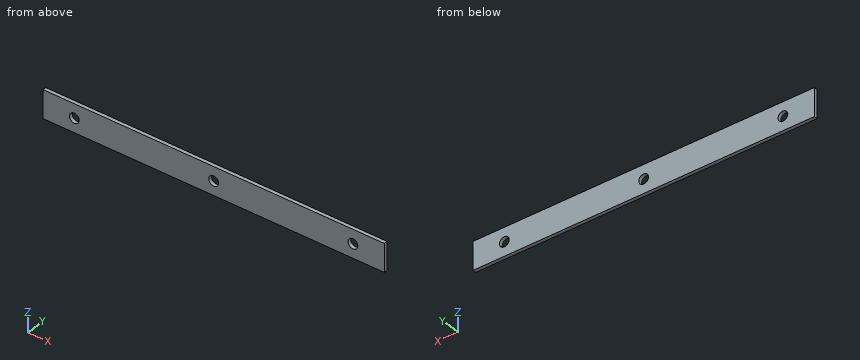
```python
from build123d import *

# Parameters (mm, degrees)
SKETCH1_W            = 245
SKETCH1_H            = 20
BASE_FLANGE1_DEPTH   = 2.5
SKETCH6_R            = 3.5
CUT_EXTRUDE1_DEPTH   = 10
LPATTERN1_COUNT      = 6
LPATTERN1_PITCH      = 146
LPATTERN1_COUNT_DIR2 = 6
LPATTERN1_PITCH_DIR2 = 146
LPATTERN2_COUNT      = 2
LPATTERN2_PITCH      = 100
LPATTERN2_COL_COUNT  = 2
LPATTERN2_COL_PITCH  = 100


# Sheet-metal steps are written as plain solids
with BuildPart() as part:
    # Sketch1 → Base-Flange1 (new body)
    with BuildSketch(Plane(origin=(0, 0, 0), x_dir=(1, 0, 0), z_dir=(0, 1, 0))):
        Rectangle(SKETCH1_W, SKETCH1_H)
    extrude(amount=-BASE_FLANGE1_DEPTH)

    # Sketch6 → Cut-Extrude1 (cut)
    with BuildSketch(Plane(origin=(0, 0, 0), x_dir=(1, 0, 0), z_dir=(0, 1, 0))):
        with Locations(Location((0, 0, 0), (0, 0, 270))):
            Circle(SKETCH6_R)
    cut_extrude1 = extrude(amount=-CUT_EXTRUDE1_DEPTH, mode=Mode.SUBTRACT)

    # LPattern1: Cut-Extrude1 6 × 6
    with Locations(*[Vector(-1, 0, 0) * (i * LPATTERN1_PITCH) + Vector(1, 0, 0) * (j * LPATTERN1_PITCH_DIR2) for i in range(LPATTERN1_COUNT) for j in range(LPATTERN1_COUNT_DIR2) if (i, j) != (0, 0)]):
        add(cut_extrude1, mode=Mode.SUBTRACT)

    # LPattern2: Cut-Extrude1 ×2
    with Locations(*[(-i * LPATTERN2_PITCH, 0, 0) for i in range(1, LPATTERN2_COUNT)]):
        add(cut_extrude1, mode=Mode.SUBTRACT)

    # LPattern2 col: Cut-Extrude1 ×2
    with Locations(*[(i * LPATTERN2_COL_PITCH, 0, 0) for i in range(1, LPATTERN2_COL_COUNT)]):
        add(cut_extrude1, mode=Mode.SUBTRACT)


solid = part.part
```
CAD build for the part. Positions are in the model's coordinates, mm. Coordinates: 2 decimals unless noted, no trailing zeros. Write each loop counter-clockwise with the first axis right and the second up, starting at its lowest first coordinate (ties: lowest second). Pieces come first, ordered by that corner, then holes.
(1) Cut at C-C, the plane y = -0.6. List the corners of the cut face in (x, z), and give its area (3 significant figures).
(2) Cut at A-A, the plane x = -100. List the corners of the cut face in (y, z), and give its area (3 significant figures).
(3) Cut at B-B, the plane z = 0. List the corners of the cut face in (x, y), and give its area (3 significant figures).
(4) Flat gauge pin, fed straight in: pin 1 (9 mm diameter, centred on x = -100, z = 0, fed in from -Y). Where does the tip first touch, or does it go through?
(5) Drill centre lines: probe 1 along X at (y, z) = (-1.65, 0); probe 2 along X at (y, z) = (-2.1, -0.75); probe 3 along Z at (x, y) = (-100.5, -2.2). Where is each one in solid material? Low to high.
Geometry says:
1. outline: (-122.5, -10) - (122.5, -10) - (122.5, 10) - (-122.5, 10) - close; hole circle Ø7 at (-100, 0); hole circle Ø7 at (0, 0); hole circle Ø7 at (100, 0)
1. area: 4,780 mm2
2. outline: (-2.5, -10) - (0, -10) - (0, -3.5) - (-2.5, -3.5) - close; (-2.5, 3.5) - (0, 3.5) - (0, 10) - (-2.5, 10) - close
2. area: 32.5 mm2
3. outline: (-122.5, -2.5) - (-103.5, -2.5) - (-103.5, 0) - (-122.5, 0) - close; (-96.5, -2.5) - (-3.5, -2.5) - (-3.5, 0) - (-96.5, 0) - close; (3.5, -2.5) - (96.5, -2.5) - (96.5, 0) - (3.5, 0) - close; (103.5, -2.5) - (122.5, -2.5) - (122.5, 0) - (103.5, 0) - close
3. area: 560 mm2
4. pin 1: stops at y = -2.5
5. probe 1: x = -122.5 to -103.5, -96.5 to -3.5, 3.5 to 96.5, 103.5 to 122.5
5. probe 2: x = -122.5 to -103.42, -96.58 to -3.42, 3.42 to 96.58, 103.42 to 122.5
5. probe 3: z = -10 to -3.46, 3.46 to 10
